Autodesk Inventor part; units mm, degrees
ref_plane "YZ Plane" through (0, 0, 0) normal (1, 0, 0) x (0, 1, 0)
ref_plane "XZ Plane" through (0, 0, 0) normal (0, 1, 0) x (-1, 0, 0)
ref_plane "XY Plane" through (0, 0, 0) normal (0, 0, 1) x (1, 0, 0)
sketch "Sketch1" plane through (0, 0, 0) normal (0, 0, 1) x (1, 0, 0)
  line L0 (2.4256, 52.3404) -> (2.4256, 12.3404)
  line L1 (12.4256, 2.3404) -> (97.4256, 2.3404)
  line L2 (142.4256, 22.3404) -> (142.4256, 52.3404)
  line L3 (127.4256, 62.3404) -> (12.4256, 62.3404)
  line L4 (2.4256, 52.3404) -> (12.4256, 62.3404)
  line L5 (97.4256, 2.3404) -> (132.4256, 12.3404)
  line L6 (2.4256, 12.3404) -> (12.4256, 2.3404)
  line L7 (142.4256, 22.3404) -> (132.4256, 12.3404)
  line L8 (127.4256, 62.3404) -> (142.4256, 52.3404)
  line L9 (12.4256, 49.8404) -> (12.4256, 47.3404)
  line L10 (63.4256, 49.8404) -> (63.4256, 47.3404)
  line L11 (12.4256, 47.3404) -> (63.4256, 47.3404)
  line L12 (63.4256, 47.3404) -> (63.4256, 49.8404)
  line L13 (63.4256, 49.8404) -> (12.4256, 49.8404)
  line L14 (12.4256, 14.8404) -> (12.4256, 17.3404)
  line L15 (63.4256, 14.8404) -> (63.4256, 17.3404)
  line L16 (12.4256, 17.3404) -> (63.4256, 17.3404)
  line L17 (63.4256, 17.3404) -> (63.4256, 14.8404)
  line L18 (63.4256, 14.8404) -> (12.4256, 14.8404)
  point P0 (0, 0)
  dimension "d14" = 140
  dimension "d15" = 10
  dimension "d16" = 10
  dimension "d17" = 51
  dimension "d18" = 51
extrude "Extrusion1" add sketch "Sketch1" against normal blind 4 contours L4 L3 L8 L2 L7 L5 L1 L6 L0 | L13 L10 L11 L9 | L14 L16 L15 L18
extrude "Extrusion2" add sketch "Sketch1" along normal blind 5.6 contours L13 L10 L11 L9 | L14 L16 L15 L18
sketch "Sketch2" plane through (12.4256, 14.8404, 5.6) normal (0, -1, 0) x (1, 0, 0)
  line L0 (0, -5.6) -> (0, 0)
  line L1 (51, -5.6) -> (51, 0)
  circle A0 centre (8.5, -2.8) radius 1.35
  circle A1 centre (25.5, -2.8) radius 1.35
  circle A2 centre (42.5, -2.8) radius 1.35
  point P0 (50.8, -5.6)
  point P1 (-12.4256, -5.6)
  dimension "d5" = 2.7
  dimension "d6" = 8.5
  dimension "d7" = 2.7
  dimension "d8" = 2.7
  dimension "d9" = 8.5
  dimension "d10" = 17
extrude "Extrusion3" cut sketch "Sketch2" against normal through all
chamfer "Chamfer1" distance 5.6 angle 45 4 edges at (12.4256, 16.0904, 5.6) (63.4256, 48.5904, 5.6) (63.4256, 16.0904, 5.6) (12.4256, 48.5904, 5.6)
properties part number "Right foot" material "Aluminum-6061"
Can you work these out from the model? Positions are in its coordinate system, mm. A direction names the side the tool comes from. Coordinates: 2 decimals unless noted, no trailing zeros. Order: outer loops, then holes, each group sorted by start corner. A loop starts at its lowest first (then second) coordinate and runs counter-clockwise, first axis right, second up.
1. For faces 1 (the face through (60.587, 16.108, 2.839)), 2 (the face through (38, 14.84, 1)), 3 (the face through (38, 17.34, 1)), which set-ups out of +Z, -Z, +X, -X, +Y, -Y let a thin tool reach every point of the face, with its end or its side?
2. If we section it at B-B (x = 45.5): Please give me the cut outline in (y, z).
3. I'm going to push flat-ended pins straight in: pin 1 (4.5 mm diameter, centred on x = 45.5, z = 3, fed in from +Y); pin 2 (3 mm diameter, centred on x = 31.5, z = 2.5, fed in from -Y); pin 3 (1.6 mm diameter, centred on x = 54.93, z = 2.8, fed in from -Y); pin 4 (18 mm diameter, centred on x = 96, y = 19, fed in from +Z). Where does each tip first touch, or does it pass through?
4. I need wall thicknesses on line 1 (Y direction, x = 47.5, z = 0.75); line 2 (Z direction, x = 55.5, y = 51.5); line 3 (X direction, y = 14.5, z = -1.5). Which ranges of each line are inside material? Lowest first, please.
5. Thinking about a two-plate mould opening in Z: for faces 4 (the face through (38, 49.84, 1)), 5 (the face through (60.587, 48.573, 2.839)), 6 (the face through (22.21, 48.57, 3.21)), which applies, +Z half, -Z half, draft (parallel to the pull), parting line (faces both ways), or undercut?
6. If we section it at D-D (x = 76): Please give me the cut outline in (y, z).
7. If we section it at A-A (z = 2.8): Give the number of separate pieces and of enclosed holes in the cut face, then the cut area to 3 significant figures.
8. If we section it at C-C (y = 36): Please give me the cut outline in (x, z), then the cut area to 3 significant figures.
Entries:
1. face 1: +Z, +X, +Y, -Y
1. face 2: +Z, +X, -X, -Y
1. face 3: +Z, +X, -X
2. outline: (2.34, -4) - (62.34, -4) - (62.34, 0) - (49.84, 0) - (49.84, 5.6) - (47.34, 5.6) - (47.34, 0) - (17.34, 0) - (17.34, 5.6) - (14.84, 5.6) - (14.84, 0) - (2.34, 0) - close
3. pin 1: stops at y = 49.84
3. pin 2: stops at y = 14.84
3. pin 3: passes through
3. pin 4: stops at z = 0
4. line 1: y = 14.84 to 17.34, 47.34 to 49.84
4. line 2: z = -4 to 0
4. line 3: x = 2.43 to 134.59
5. face 4: draft
5. face 5: +Z half
5. face 6: undercut
6. outline: (2.34, -4) - (62.34, -4) - (62.34, 0) - (2.34, 0) - close
7. separate pieces: 8
7. enclosed holes: 0
7. area: 187 mm2
8. outline: (2.43, -4) - (142.43, -4) - (142.43, 0) - (2.43, 0) - close
8. area: 560 mm2
